Design review of the part shown in the three views and the two pictorial views. Dimensions are in mm from the part's minimum x, y and z. A direction names the side the tool comes from. Coordinates: 2 decimals unless noted, no trailing zeros. Loops run counter-clockwise (first coordinate to the right, second up) from the corner with the lowest first, then second, coordinate; pieces in that order, holes last. Notation, with made-up numbers: (34.25, -19) -> (52.25, -19) arc R27 cw to (52.25, -2) -> close; hole circle Ø5 at (3.5, 6.25). An arc over 180 degrees is marked (long way). One line per item, written item: value.
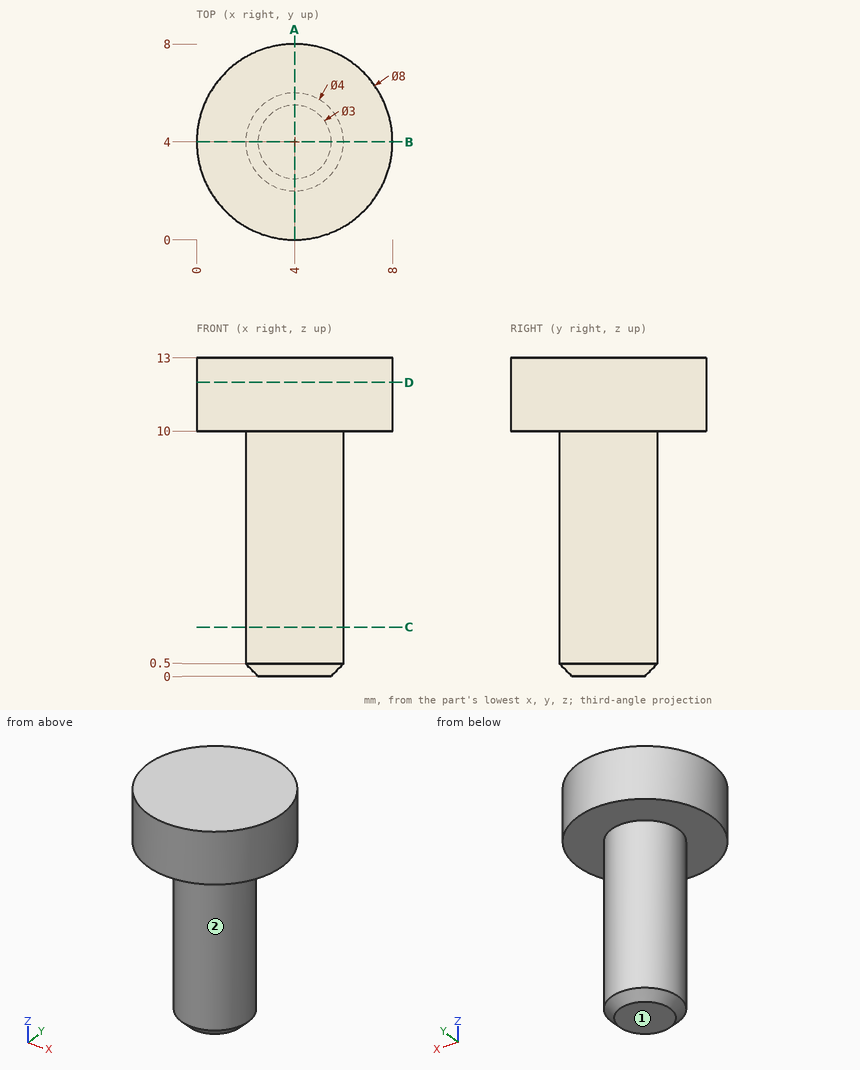
1. Insertion check: pin 1 Ø1.5 at (y, z) = (4.5, 9) entering from -X; pin 2 Ø4 at (x, z) = (6.5, 10) entering from +Y. Each pin has a flat end and moves straight along its axis. Give the tip position at first contact, or say it passes through.
Return value:
pin 1: stops at x = 2
pin 2: stops at y = 7.97
2. For the marked faces 1 and 2, list the 3-axis set-ups (+Z, -Z, +X, -X, +Y, -Y) from which the entire face can be reached by the end or side of a thin tool; tool diameter is ignored.
Return value:
face 1: -Z, +X, -X, +Y, -Y
face 2: -Z
3. Take a section at D-D, the plane z = 12. Give the boundary of the cut face in (x, y), and give its area (3 significant figures).
Return value:
outline: circle Ø8 at (4, 4)
area: 50.3 mm2
4. To check wall thickness, follow probe 1 along Z at (x, y) = (0.75, 4.75); probe 2 along Y at (x, z) = (2.5, 3.25); probe 3 along Y at (x, z) = (4.25, 7.5). State the ranges of each line that lie inside material, in increasing order. Write a range as from..to.
Return value:
probe 1: z = 10..13
probe 2: y = 2.68..5.32
probe 3: y = 2.02..5.98
5. Take a section at C-C, the plane z = 2. Give the boundary of the cut face in (x, y), and give its area (3 significant figures).
Return value:
outline: circle Ø4 at (4, 4)
area: 12.6 mm2
6. Take a section at A-A, the plane x = 4. Give the boundary of the cut face in (y, z).
Return value:
outline: (0, 10) -> (2, 10) -> (2, 0.5) -> (2.5, 0) -> (5.5, 0) -> (6, 0.5) -> (6, 10) -> (8, 10) -> (8, 13) -> (0, 13) -> close
